Drawing for the job (mm, zero at the part's lowest x, y, z). A direction names the side the tool comes from. Coordinates: 2 decimals unless noted, no trailing zeros. Order: outer loops, then holes, each group sorted by start corner. A loop starts at its lowest first (then second) coordinate and runs counter-clockwise, first axis right, second up. Notation, with made-up numbers: (68, 13.5) -> (96, 13.5) arc R10 ccw to (96, 26.5) -> close; hole circle Ø7 at (66.5, 8.25). An arc over 180 degrees is marked (long way). Write each question's results on one line, items separated by ' | '.
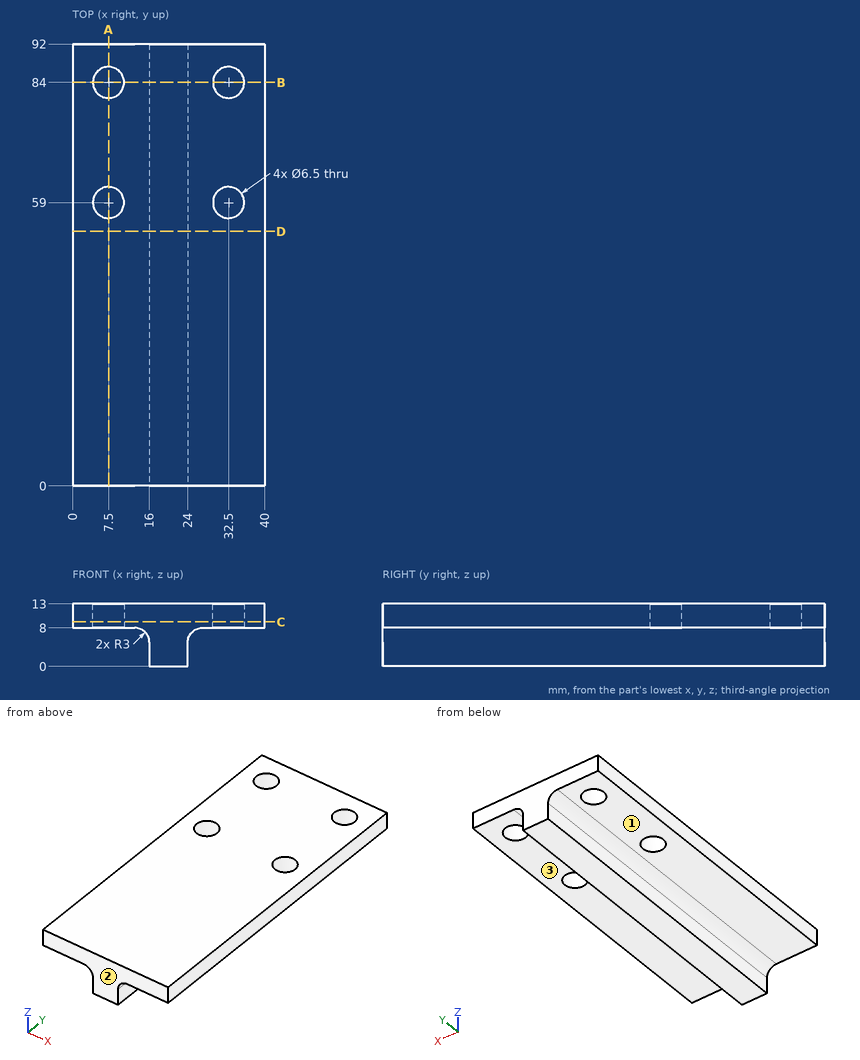
Item 1: Slice it at B-B, the plane y = 84. List the corners of the cut face in (x, z).
Answer:
outline: (0, 8) -> (4.25, 8) -> (4.25, 13) -> (0, 13) -> close; (10.75, 8) -> (13, 8) arc R3 cw to (16, 5) -> (16, 0) -> (24, 0) -> (24, 5) arc R3 cw to (27, 8) -> (29.25, 8) -> (29.25, 13) -> (10.75, 13) -> close; (35.75, 8) -> (40, 8) -> (40, 13) -> (35.75, 13) -> close
Item 2: Pin check, flat tips, straight feed: pin 1 (4 mm diameter, centred on y = 56, z = 1.5, fed in from -X); pin 2 (5 mm diameter, centred on y = 39, z = 7.5, fed in from -X); pin 3 (1.5 mm diameter, centred on y = 43.5, z = 3, fed in from +X); pin 4 (8.5 mm diameter, centred on x = 7.5, y = 84, fed in from -Z). Stop position of each tip, or through.
Answer:
pin 1: stops at x = 16 | pin 2: stops at x = 0 | pin 3: stops at x = 24 | pin 4: stops at z = 8
Item 3: Tool access for the marked faces 1, 2 and 3: list every direction of +Z, -Z, +X, -X, +Y, -Y with a clear straight run to the whole face (end or side of a thin tool).
Answer:
face 1: -Z, -X, +Y, -Y | face 2: +Z, -Z, +X, -X, -Y | face 3: -Z, +X, +Y, -Y
Item 4: Drill centre lines: line 1 (Y direction, x = 32.5, z = 11.15); line 2 (Z direction, x = 9.5, y = 66); line 3 (X direction, y = 84.5, z = 9). Where is each one in solid material? Low to high. Write a range as from..to.
Answer:
line 1: y = 0..55.75, 62.25..80.75, 87.25..92 | line 2: z = 8..13 | line 3: x = 0..4.29, 10.71..29.29, 35.71..40
Item 5: Slice it at D-D, the plane y = 53. List the corners of the cut face in (x, z), and give its area (3 significant figures).
Answer:
outline: (0, 8) -> (13, 8) arc R3 cw to (16, 5) -> (16, 0) -> (24, 0) -> (24, 5) arc R3 cw to (27, 8) -> (40, 8) -> (40, 13) -> (0, 13) -> close | area: 268 mm^2
Item 6: Slice it at C-C, the plane z = 9.25. List the corners of the cut face in (x, y), and give its area (3 significant figures).
Answer:
outline: (0, 0) -> (40, 0) -> (40, 92) -> (0, 92) -> close; hole circle Ø6.5 at (7.5, 59); hole circle Ø6.5 at (7.5, 84); hole circle Ø6.5 at (32.5, 59); hole circle Ø6.5 at (32.5, 84) | area: 3,550 mm^2
Item 7: Slice it at A-A, the plane x = 7.5. List the corners of the cut face in (y, z), and give its area (3 significant figures).
Answer:
outline: (0, 8) -> (55.75, 8) -> (55.75, 13) -> (0, 13) -> close; (62.25, 8) -> (80.75, 8) -> (80.75, 13) -> (62.25, 13) -> close; (87.25, 8) -> (92, 8) -> (92, 13) -> (87.25, 13) -> close | area: 395 mm^2
